from build123d import *

# Parameters (mm, degrees)
SKETCH1_W           = 304.8
SKETCH1_H           = 660.4
SKETCH1_R           = 16.8275
SKETCH1_R_2         = 2.2479
BOSS_EXTRUDE1_DEPTH = 3.175


with BuildPart() as part:
    # Sketch1 → Boss-Extrude1 (new body)
    with BuildSketch(Plane(origin=(0, 0, 0), x_dir=(1, 0, 0), z_dir=(0, 1, 0))):
        with Locations((152.4, 330.2)):
            Rectangle(SKETCH1_W, SKETCH1_H)
        with Locations(Location((46.0248, 330.2, 0), (0, 0, 270))):
            Circle(SKETCH1_R, mode=Mode.SUBTRACT)
        with Locations(Location((258.7752, 330.2, 0), (0, 0, 270))):
            Circle(SKETCH1_R, mode=Mode.SUBTRACT)
        with Locations(Location((29.633333333, 19.05, 0), (0, 0, 270))):
            Circle(SKETCH1_R_2, mode=Mode.SUBTRACT)
        with Locations(Location((59.266666667, 19.05, 0), (0, 0, 270))):
            Circle(SKETCH1_R_2, mode=Mode.SUBTRACT)
        with Locations(Location((245.533333333, 19.05, 0), (0, 0, 270))):
            Circle(SKETCH1_R_2, mode=Mode.SUBTRACT)
        with Locations(Location((275.166666667, 19.05, 0), (0, 0, 270))):
            Circle(SKETCH1_R_2, mode=Mode.SUBTRACT)
        with Locations(Location((275.166666667, 641.35, 0), (0, 0, 270))):
            Circle(SKETCH1_R_2, mode=Mode.SUBTRACT)
        with Locations(Location((245.533333333, 641.35, 0), (0, 0, 270))):
            Circle(SKETCH1_R_2, mode=Mode.SUBTRACT)
        with Locations(Location((59.266666667, 641.35, 0), (0, 0, 270))):
            Circle(SKETCH1_R_2, mode=Mode.SUBTRACT)
        with Locations(Location((29.633333333, 641.35, 0), (0, 0, 270))):
            Circle(SKETCH1_R_2, mode=Mode.SUBTRACT)
    extrude(amount=BOSS_EXTRUDE1_DEPTH)


solid = part.part
Can you work these out from the model? Positions are in its coordinate system, mm. Coordinates: 2 decimals unless noted, no trailing zeros. Order: outer loops, then holes, each group sorted by start corner. A loop starts at its lowest first (then second) coordinate and runs counter-clockwise, first axis right, second up. Notation, with made-up numbers: (-7.5, 57) - (3.5, 57) arc R34 ccw to (3.5, 87) - close; hole circle Ø4 at (89.5, 67.25). An arc over 180 degrees is marked (long way). Answer as a JSON object with one key per item and string values. Group by question number.
Q1. We'd pull the mould along X, two halves only. Please class faces 1 (the face through (150, 0, -335)), 2 (the face through (39.58, 1.565, -314.656)), 3 (the face through (252.33, 1.565, -314.656)): +X half, -X half, draft (parallel to the pull), parting line (faces both ways), or undercut.
Q2. Imagine slicing it at A-A (z = -330.2). Please give me the cut outline in (x, y) (3 decimals), and give its area (3 significant figures).
Q3. I need wall thicknesses on line 1 (X direction, y = 1, z = -641.35); line 2 (X direction, y = 1.75, z = -330.2); line 3 (X direction, y = 2.9, z = -316). Which ranges of each line are inside material? Lowest first, please. Write a range as from..to.
Determined:
{
 "1": {"face 1": "draft", "face 2": "undercut", "face 3": "undercut"},
 "2": {"outline": "(0, 0) - (29.197, 0) - (29.197, 3.175) - (0, 3.175) - close; (62.852, 0) - (241.948, 0) - (241.948, 3.175) - (62.852, 3.175) - close; (275.603, 0) - (304.8, 0) - (304.8, 3.175) - (275.603, 3.175) - close", "area": "754 mm2"},
 "3": {"line 1": "x = 0..27.39, 31.88..57.02, 61.51..243.29, 247.78..272.92, 277.41..304.8", "line 2": "x = 0..29.2, 62.85..241.95, 275.6..304.8", "line 3": "x = 0..37, 55.05..249.75, 267.8..304.8"}
}
